Work out the finished part from the listing and answer in its coordinate system (mm). A direction names the side the tool comes from. Give positions to 0.01 mm unless a question says otherwise; leave off trailing zeros. Loops run counter-clockwise (first coordinate to the right, second up) from the corner with the lowest first, then second, coordinate; pieces in that order, holes last. Notation, with made-up numbers: (-7, 16) - (34, 16) arc R13 ccw to (34, 33) - close; hole circle Ø9 at (63, 23). An arc over 180 degrees is marked (long way). Use CSV: the item, a comma, the result in double quotes.
from build123d import *

# Parameters (mm, degrees)
F0_W     = 127
F0_H     = 304.8
F0_R     = 13.716
F1_DEPTH = 5.08


with BuildPart() as f1:
    # F0 (on Front) → F1 (new body)
    with BuildSketch(Plane.XZ):
        with Locations((63.5, -152.4)):
            Rectangle(F0_W, F0_H)
        with BuildLine():
            Line((95.25, -266.7), (31.75, -266.7))
            Line((31.75, -266.7), (31.75, -247.65))
            ThreePointArc((31.75, -247.65), (37.329616, -234.179616), (50.8, -228.6))
            Line((50.8, -228.6), (76.2, -228.6))
            ThreePointArc((76.2, -228.6), (89.670384, -234.179616), (95.25, -247.65))
            Line((95.25, -247.65), (95.25, -266.7))
        make_face(mode=Mode.SUBTRACT)
        with Locations((63.5, -38.1)):
            Circle(F0_R, mode=Mode.SUBTRACT)
    extrude(amount=F1_DEPTH)


solid = f1.part
Item 1: A cutting plane is placed at A-A on x = 63.5. Determine the outline of the cut face in (y, z), and give its area (3 significant figures).
Determined:
outline,"(-5.08, -304.8) - (0, -304.8) - (0, -266.7) - (-5.08, -266.7) - close; (-5.08, -228.6) - (0, -228.6) - (0, -51.82) - (-5.08, -51.82) - close; (-5.08, -24.38) - (0, -24.38) - (0, 0) - (-5.08, 0) - close"
area,"1,220 mm²"
Item 2: A cutting plane is placed at B-B on z = -38.1. Determine the outline of the cut face in (x, y), and give its area (3 significant figures).
Determined:
outline,"(0, -5.08) - (49.78, -5.08) - (49.78, 0) - (0, 0) - close; (77.22, -5.08) - (127, -5.08) - (127, 0) - (77.22, 0) - close"
area,"506 mm²"
Item 3: A cutting plane is placed at D-D on z = -258.5. Determine the outline of the cut face in (x, y), and give its area (3 significant figures).
Determined:
outline,"(0, -5.08) - (31.75, -5.08) - (31.75, 0) - (0, 0) - close; (95.25, -5.08) - (127, -5.08) - (127, 0) - (95.25, 0) - close"
area,"323 mm²"
Item 4: For faces 1 (the flat face through (95.25, -3, -257)), 2 (the flat face through (63, -3, -304.8)), determine the directions among +Z, -Z, +X, -X, +Y, -Y from which every point of the face is accessible in a straight line to the end or side of a thin tool.
Determined:
face 1,"+Y, -Y"
face 2,"-Z, +X, -X, +Y, -Y"
Item 5: A cutting plane is placed at C-C on y = -3.4. Determine the outline of the cut face in (x, z), and give its area (3 significant figures).
Determined:
outline,"(0, -304.8) - (127, -304.8) - (127, 0) - (0, 0) - close; hole (31.75, -266.7) - (95.25, -266.7) - (95.25, -247.65) arc R19.05 ccw to (76.2, -228.6) - (50.8, -228.6) arc R19.05 ccw to (31.75, -247.65) - close; hole circle Ø27.43 at (63.5, -38.1)"
area,"35,900 mm²"
Item 6: Find the intervals of material crossed by line 1 (Z direction, x = 63.5, y = -1.15); line 2 (X direction, y = -4.7, z = -249); line 3 (X direction, y = -1.45, z = -245), in increasing order.
Determined:
line 1,"z = -304.8 to -266.7, -228.6 to -51.82, -24.38 to 0"
line 2,"x = 0 to 31.75, 95.25 to 127"
line 3,"x = 0 to 31.94, 95.06 to 127"
Item 7: Given P1, Ø10, axis at x = 41.5, z = -241.5, coming from the +Y side, flat-ended and moving along its own axis, determine where the tip first touches the part or whether it passes through.
Determined:
P1,"passes through"
